```python
from build123d import *

# Parameters (mm, degrees)
EXTRUDE_THIN1_DEPTH = 9.5
FILLET1_R           = 1
FILLET2_R           = 0.2
CUT_EXTRUDE1_DEPTH  = 2


with BuildPart() as part:
    # Sketch1 → Extrude-Thin1 (new body, symmetric)
    with BuildSketch(Plane(origin=(0, 0, 0), x_dir=(1, 0, 0), z_dir=(0, 1, 0))):
        Polygon((-0.5, 0), (-0.5, -37.779994735), (-33.810186195, -68.303156757), (-33.134595987, -69.040434094), (0.5, -38.220005265), (0.5, 0), align=None)
    extrude(amount=EXTRUDE_THIN1_DEPTH, both=True)

    # Fillet1
    fillet1_edges = [part.edges().sort_by_distance(p)[0] for p in [
        (-0.5, 0, 37.779994735),
        (0.5, 0, 38.220005265),
    ]]
    fillet(fillet1_edges, radius=FILLET1_R)

    # Fillet2
    fillet2_edges = [part.edges().sort_by_distance(p)[0] for p in [
        (-33.810186195, 0, 68.303156757),
        (-0.5, 0, 0),
        (0.5, 0, 0),
        (-33.134595987, 0, 69.040434094),
    ]]
    fillet(fillet2_edges, radius=FILLET2_R)

    # Sketch2 → Cut-Extrude1 (cut, through all)
    with BuildSketch(Plane.ZY.offset(0.5)):
        with BuildLine():
            Line((5, 2.6), (30, 2.6))
            ThreePointArc((30, 2.6), (32.6, 0), (30, -2.6))
            Line((30, -2.6), (5, -2.6))
            ThreePointArc((5, -2.6), (2.4, 0), (5, 2.6))
        make_face()
    extrude(amount=-CUT_EXTRUDE1_DEPTH, mode=Mode.SUBTRACT)


solid = part.part
```
The listing builds one solid part. Answer for the finished solid, in the listing's coordinates (mm). Give positions to 0.01 mm unless a question says otherwise; leave off trailing zeros. Write each loop counter-clockwise with the first axis right and the second up, starting at its lowest first coordinate (ties: lowest second). Pieces come first, ordered by that corner, then holes. Notation, with made-up numbers: (58, -36.5) -> (74, -36.5) arc R25 cw to (74, -21.5) -> close; hole circle Ø5 at (-9, 25.5). An arc over 180 degrees is marked (long way). Use one line per item in the form item = value.
1) Section D-D on z = 12 is taken. Write down the section's boundary in (x, y).
Result:
outline = (-0.5, -9.5) -> (0.5, -9.5) -> (0.5, -2.6) -> (-0.5, -2.6) -> close; (-0.5, 2.6) -> (0.5, 2.6) -> (0.5, 9.5) -> (-0.5, 9.5) -> close
2) Section A-A on z = 31 is taken. Write down the section's boundary in (x, y), plus the area to 3 significant figures.
Result:
outline = (-0.5, -9.5) -> (0.5, -9.5) -> (0.5, -2.4) -> (-0.5, -2.4) -> close; (-0.5, 2.4) -> (0.5, 2.4) -> (0.5, 9.5) -> (-0.5, 9.5) -> close
area = 14.2 mm²
3) Section B-B on y = 0 is taken. Write down the section's boundary in (x, z).
Result:
outline = (-33.68, 68.45) arc R0.2 ccw to (-33.66, 68.17) -> (-0.82, 38.08) arc R1 cw to (-0.5, 37.34) -> (-0.5, 32.6) -> (0.5, 32.6) -> (0.5, 37.78) arc R1 ccw to (0.18, 38.52) -> (-32.99, 68.91) arc R0.2 ccw to (-33.27, 68.89) -> close; (-0.5, 0.2) arc R0.2 ccw to (-0.3, 0) -> (0.3, 0) arc R0.2 ccw to (0.5, 0.2) -> (0.5, 2.4) -> (-0.5, 2.4) -> close
4) Section C-C on y = 4.5 is taken. Write down the section's boundary in (x, z), plus the area to 3 significant figures.
Result:
outline = (-33.68, 68.45) arc R0.2 ccw to (-33.66, 68.17) -> (-0.82, 38.08) arc R1 cw to (-0.5, 37.34) -> (-0.5, 0.2) arc R0.2 ccw to (-0.3, 0) -> (0.3, 0) arc R0.2 ccw to (0.5, 0.2) -> (0.5, 37.78) arc R1 ccw to (0.18, 38.52) -> (-32.99, 68.91) arc R0.2 ccw to (-33.27, 68.89) -> close
area = 83.4 mm²
5) Straight lines are drawn through the part: probe 1 along X at (y, z) = (6.75, 36.5); probe 2 along Z at (x, y) = (-12, -1); probe 3 along Z at (x, y) = (-7.5, 7.75). For each, find the intervals that lie inside material, in ascending order.
Result:
probe_1 = -0.5 to 0.5
probe_2 = 48.32 to 49.67
probe_3 = 44.19 to 45.55
6) Each of these flat-tipped pins is pushed along its axis until it touches: P1, Ø5, axis at x = -28, y = -1.5, coming from the -Z side; P2, Ø9.5, axis at y = 4, z = 14.5, coming from the -X side; P3, Ø5, axis at y = -4.5, z = 39, coming from the -X side. Where does it stop, or does it pass through?
Result:
P1 = 60.69
P2 = -0.5
P3 = -4.56
7) For a pull along Y with two mould halves and no side action, classify faces 1 (the flat face through (-0.5, 4, 19)), 2 (the cylindrical face through (0, 0.1, 32.6)), 3 (the cylindrical face through (0, -0.1, 2.4)), 4 (the flat face through (-4, 9.5, 42)) as +Y half, -Y half, draft (parallel to the pull), parting line (faces both ways), or undercut.
Result:
face_1 = draft
face_2 = undercut
face_3 = undercut
face_4 = +Y half
